Part print with two shaded views. Sizes in mm from the minimum x, y, z corner. A direction names the side the tool comes from. Give positions to 0.01 mm unless a question says otherwise; leave off trailing zeros. Write each loop counter-clockwise with the first axis right and the second up, starting at its lowest first coordinate (ties: lowest second). Pieces come first, ordered by that corner, then holes. Notation, with made-up numbers: (48, 13.5) - (67, 13.5) arc R9 ccw to (67, 26.5) - close; hole circle Ø2 at (22.5, 42). An arc over 180 degrees is marked (long way). Answer as a JSON object with one key per item and string values.
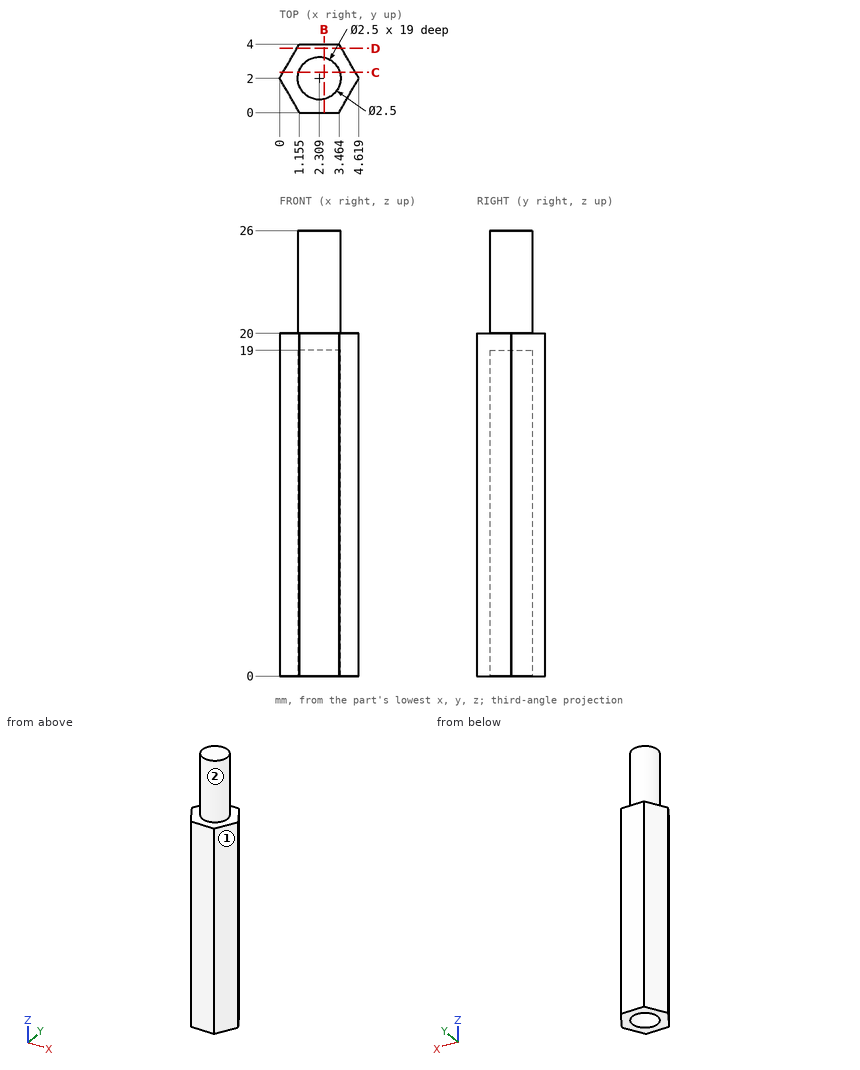
(1) Saw through at D-D, the plane y = 3.75. Give the cut face in (x, z).
Answer key:
{"outline": "(1.01, 0) - (3.61, 0) - (3.61, 20) - (1.01, 20) - close"}
(2) 3-axis set-ups, long thin cutter, end or side, ignore diameter. For the marked faces 1 and 2: which of +Z, -Z, +X, -X, +Y, -Y reach the whole face in a straight line?
Answer key:
{"face 1": "+Z, -Z, +X, -Y", "face 2": "+Z"}
(3) Saw through at C-C, the plane y = 2.35. Give the cut face in (x, z).
Answer key:
{"outline": "(0.2, 0) - (1.11, 0) - (1.11, 19) - (3.51, 19) - (3.51, 0) - (4.42, 0) - (4.42, 20) - (3.51, 20) - (3.51, 26) - (1.11, 26) - (1.11, 20) - (0.2, 20) - close"}
(4) Saw through at B-B, the plane x = 2.6. Give the cut face in (y, z) (1 decimal).
Answer key:
{"outline": "(0, 0) - (0.8, 0) - (0.8, 19) - (3.2, 19) - (3.2, 0) - (4, 0) - (4, 20) - (3.2, 20) - (3.2, 26) - (0.8, 26) - (0.8, 20) - (0, 20) - close"}
(5) Probe L1, parallel to Z at x = 2.85, y = 2; L2, parallel to Z at x = 0.65, y = 1.2; L3, parallel to Y at x = 3.1, z = 10.5. List the from-to ranges inside material, lowest first. Write a range as [from, to].
Answer key:
{"L1": "z = [19, 26]", "L2": "z = [0, 20]", "L3": "y = [0, 1.03], [2.97, 4]"}
(6) Flat gauge pin, fed straight in: P1, Ø2, axis at x = 3, y = 2.5, coming from the -Z side. Where does the tip first touch, or does it go through?
Answer key:
{"P1": "stops at z = 0"}
